Can you work these out from the model? Positions are in its coordinate system, mm. Face numbers are marked on the shaded views. A direction names the side the tool comes from. Round coordinates to 2 decimals unless told otherwise and drop trailing zeros. Loops run counter-clockwise (first coordinate to the right, second up) from the corner with the lowest first, then second, coordinate; pieces in that order, holes last. Notation, with made-up numbers: (65.25, 32.25) -> (92.25, 32.25) arc R11 cw to (92.25, 40.25) -> close; hole circle Ø4 at (10, -36). An arc over 180 degrees is marked (long way). Answer as a JSON object with one key per item and string values.
```python
from build123d import *

# Parameters (mm, degrees)
MOTOR_SHAFT_DEPTH  = 13
SKETCH4_R          = 1.5
CUT_EXTRUDE2_DEPTH = 17.5
FILLET1_R          = 2


with BuildPart() as part:
    # Sketch2 → Revolve1 (revolve)
    with BuildSketch(Plane.XY, mode=Mode.PRIVATE) as revolve1_sk:
        Polygon((13, 14), (13, 19), (15, 19), (15, 0), (-15, 0), (-15, 19), (-13, 19), (-13, 14), (-2, 7), (2, 7), align=None)
    revolve(revolve1_sk.sketch.rotate(Axis((0, 0, 0), (1, 0, 0)), 90), axis=Axis((0, 0, 0), (1, 0, 0)))

    # Sketch3 → motor shaft (cut)
    with BuildSketch(Plane.ZY.offset(15)):
        with BuildLine():
            Line((2.9, 1.574801575), (2.9, -1.574801575))
            ThreePointArc((2.9, -1.574801575), (-3.3, 0), (2.9, 1.574801575))
        make_face()
    extrude(amount=-MOTOR_SHAFT_DEPTH, mode=Mode.SUBTRACT)

    # Sketch4 → Cut-Extrude2 (cut, symmetric)
    with BuildSketch(Plane.XY):
        Circle(SKETCH4_R)
        with Locations(Location((5, 0, 0), (0, 0, 3.47e-07))):
            Circle(SKETCH4_R)
        with Locations((-5, 0)):
            Circle(SKETCH4_R)
    extrude(amount=CUT_EXTRUDE2_DEPTH, both=True, mode=Mode.SUBTRACT)

    # Fillet1
    fillet1_edges = [part.edges().sort_by_distance(p)[0] for p in [
        (13, 0, -14),
        (-13, 0, -14),
    ]]
    fillet(fillet1_edges, radius=FILLET1_R)


solid = part.part
```
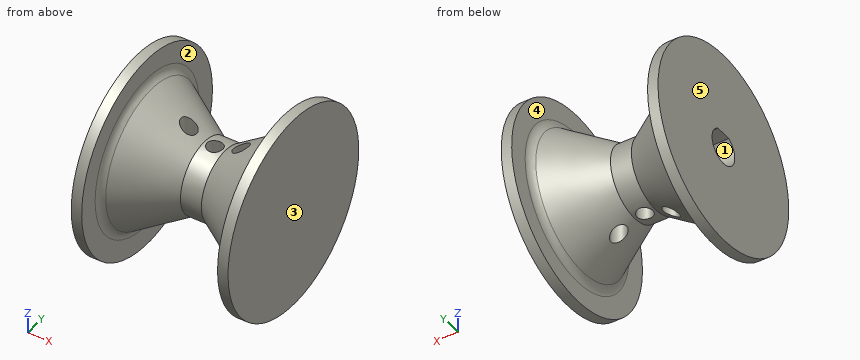
Q1. On a 3-axis mill with a long thin cutter (end or side, diameter ignored), from which of +Z, -Z, +X, -X, +Y, -Y can I reach the whole of each face in a straight line? I mean the marked faces 1 and 2. Say none if no direction works.
Determined:
{"face 1": "-X", "face 2": "none"}
Q2. I want a section at C-C, the plane x = 0. Write out the boundary of the cut face in (y, z), then the cut area to 3 significant figures.
Determined:
{"outline": "(-1.5, -6.84) -> (-1.5, 6.84) arc R7 ccw to start; (1.5, -6.84) arc R7 ccw to (1.5, 6.84) -> close", "area": "112 mm²"}
Q3. We'd pull the mould along X, two halves only. Please class the marked faces 3, 4 and 5: pulls with the +X half, pulls with the -X half, needs draft (parallel to the pull), parting line crosses it, or undercut.
Determined:
{"face 3": "pulls with the +X half", "face 4": "undercut", "face 5": "pulls with the -X half"}
Q4. I want a section at D-D, the plane x = 5. Write out the boundary of the cut face in (y, z).
Determined:
{"outline": "(-1.5, -8.78) -> (-1.5, 8.78) arc R8.91 ccw to start; (1.5, -8.78) arc R8.91 ccw to (1.5, 8.78) -> close"}
Q5. I'm going to push flat-ended pins straight in: pin 1 (8 mm diameter, centred on x = 11, y = 14.5, fed in from -Z); pin 2 (0.9 mm diameter, centred on x = -8, y = 0, fed in from -Z); pin 3 (2 mm diameter, centred on x = 3, z = 3.5, fed in from -Y). Where does each tip first touch, or does it pass through?
Determined:
{"pin 1": "z = -15.47", "pin 2": "z = -11.1", "pin 3": "y = -7.62"}
Q6. I want a section at A-A, the plane x = -5. Write out the boundary of the cut face in (y, z), then the cut area to 3 significant figures.
Determined:
{"outline": "(-1.57, 2.9) -> (-1.5, 2.9) -> (-1.5, 8.78) arc R8.91 ccw to (-1.5, -8.78) -> (-1.5, -2.94) arc R3.3 cw to start; (1.5, -8.78) arc R8.91 ccw to (1.5, 8.78) -> (1.5, 2.9) -> (1.57, 2.9) arc R3.3 cw to (1.5, -2.94) -> close", "area": "181 mm²"}
Q7. If I drill on L1, parallel to X at y = 16, z = 6.5; L2, parallel to X at y = -0.5, z = -6.5; L3, parallel to X at y = -11, z = 1, over which ranges is the centre line in solid material (lowest first)? Write a range as [from, to].
Determined:
{"L1": "[-15, -13], [13, 15]", "L2": "[-15, -6.41], [-3.59, -1.41], [1.41, 3.59], [6.41, 15]", "L3": "[-15, -8.36], [8.36, 15]"}
Q8. I want a section at B-B, the plane z = -1. Give the number of separate pieces and of enclosed holes in the cut face, then the cut area to 3 significant figures.
Determined:
{"separate pieces": "1", "enclosed holes": "2", "area": "572 mm²"}
